from build123d import *

# Parameters (mm, degrees)
CYLINDER001_R     = 8.4
CYLINDER001_DEPTH = 5.5
CYLINDER004_R     = 7.2
CYLINDER004_DEPTH = 6.5
CYLINDER003_R     = 10.4
CYLINDER003_DEPTH = 1
CYLINDER002_R     = 10.4
CYLINDER002_DEPTH = 2.75
SKETCH013_R       = 9.6
SKETCH013_R_2     = 2.2
PAD011_DEPTH      = 3.75


with BuildPart() as bearing_holder_extract:
    # Cylinder001 → Cylinder001 (new body)
    with BuildSketch(Plane.XY):
        Circle(CYLINDER001_R)
    extrude(amount=CYLINDER001_DEPTH)


with BuildPart() as bearing_holder_extract_fusion:
    # Cylinder004 → Cylinder004 (new body)
    with BuildSketch(Plane.XY.offset(-1)):
        Circle(CYLINDER004_R)
    extrude(amount=CYLINDER004_DEPTH)

    # Fusion001: union bearing holder extract
    add(bearing_holder_extract.part)


with BuildPart() as bearing_holder_disk:
    # Cylinder003 → Cylinder003 (new body)
    with BuildSketch(Plane.XY.offset(-1)):
        Circle(CYLINDER003_R)
    extrude(amount=CYLINDER003_DEPTH)


with BuildPart() as bearing_holder_body:
    # Cylinder002 → Cylinder002 (new body)
    with BuildSketch(Plane.XY):
        Circle(CYLINDER002_R)
    extrude(amount=CYLINDER002_DEPTH)

    # Fusion002: union bearing holder disk
    add(bearing_holder_disk.part)

    # Cut003: cut bearing holder extract fusion
    add(bearing_holder_extract_fusion.part, mode=Mode.SUBTRACT)


with BuildPart() as bearing_holder_body_1:
    # Cut003 placement: moved
    add(bearing_holder_body.part.moved(Location((0, 0, 1))))


with BuildPart() as bearing_holder_body_clone:
    # Body009 base: copy of bearing holder body
    add(bearing_holder_body_1.part)


with BuildPart() as bearing_holder_body_clone_1:
    # Clone002 placement: moved
    add(bearing_holder_body_clone.part.moved(Location((0, 0, -1))))


with BuildPart() as bearing_holder_body_clone_2:
    # Body009 placement: moved
    add(bearing_holder_body_clone_1.part.moved(Location((10, 25, 1))))


with BuildPart() as bearing_holder_body_clone001:
    # Body010 base: copy of bearing holder body
    add(bearing_holder_body_1.part)


with BuildPart() as bearing_holder_body_clone001_1:
    # Clone003 placement: moved
    add(bearing_holder_body_clone001.part.moved(Location((0, 0, -1))))


with BuildPart() as bearing_holder_body_clone001_2:
    # Body010 placement: moved
    add(bearing_holder_body_clone001_1.part.moved(Location((-26, -20, 1))))


with BuildPart() as bearing_holder_body_clone002:
    # Body011 base: copy of bearing holder body
    add(bearing_holder_body_1.part)


with BuildPart() as bearing_holder_body_clone002_1:
    # Clone004 placement: moved
    add(bearing_holder_body_clone002.part.moved(Location((0, 0, -1))))


with BuildPart() as bearing_holder_body_clone002_2:
    # Body011 placement: moved
    add(bearing_holder_body_clone002_1.part.moved(Location((46, -20, 1))))


with BuildPart() as top_bearing_plate_fusion_clone:
    # Sketch013 → Pad011 (new body)
    with BuildSketch(Plane.XY):
        with BuildLine():
            Line((1.646601, 32.001411), (-34.644004, -12.858892))
            ThreePointArc((-34.644004, -12.858892), (-36.048496, -24.763041), (-25.91021, -31.158079))
            Line((-25.91021, -31.158079), (45.861431, -31.158079))
            ThreePointArc((45.861431, -31.158079), (55.920577, -24.833853), (54.581009, -13.027591))
            Line((54.581009, -13.027591), (18.635324, 31.950884))
            ThreePointArc((18.635324, 31.950884), (10.153066, 36.045837), (1.646601, 32.001411))
        make_face()
        with Locations((-25.91021, -19.924263)):
            Circle(SKETCH013_R, mode=Mode.SUBTRACT)
        with Locations((10.120649, 25.146166)):
            Circle(SKETCH013_R, mode=Mode.SUBTRACT)
        with Locations((45.861431, -19.996062)):
            Circle(SKETCH013_R, mode=Mode.SUBTRACT)
        with Locations((-11.219142, 6.834813)):
            Circle(SKETCH013_R_2, mode=Mode.SUBTRACT)
        with Locations((10.016696, -25.022005)):
            Circle(SKETCH013_R_2, mode=Mode.SUBTRACT)
        with Locations((31.129337, 6.879182)):
            Circle(SKETCH013_R_2, mode=Mode.SUBTRACT)
    extrude(amount=PAD011_DEPTH)

    # Fusion003: union bearing holder body clone, bearing holder body clone001, bearing holder body clone002
    add(bearing_holder_body_clone_2.part)
    add(bearing_holder_body_clone001_2.part)
    add(bearing_holder_body_clone002_2.part)


with BuildPart() as top_bearing_plate_fusion_clone_1:
    # Body021 placement: moved
    add(top_bearing_plate_fusion_clone.part.moved(Location((-10, -8, 0))))


solid = top_bearing_plate_fusion_clone_1.part
For this review, take the finished solid that the model builds, in its own axes (mm). A direction names the side the tool comes from. Round coordinates to 2 decimals unless told otherwise and drop trailing zeros. Write each loop counter-clockwise with the first axis right and the second up, starting at its lowest first coordinate (ties: lowest second). Pieces come first, ordered by that corner, then holes. Notation, with made-up numbers: (75.25, 66.25) - (123.25, 66.25) arc R13 ccw to (123.25, 75.25) - close; hole circle Ø10 at (-29.5, -39). An arc over 180 degrees is marked (long way). Write item = value, one per line. Start each with the question number.
1. Draft analysis for pull direction X (two halves, no side actions). For faces 1 (the face through (-26.24, 1.89, 1.85)), 2 (the face through (45.843, -32.991, 1.849)), 3 (the face through (-43.193, -27.683, 0.493)), state which applies: released by +X, released by -X, zero draft, split by the parting line, or undercut.
2. Wall thickness on L1, parallel to X at y = -28, z = 2.25; L2, parallel to X at y = -28, z = 0.5; L3, parallel to X at y = -33, z = 1.55: over which ranges is each line inside the solid? List them lowest first.
3. For faces 4 (the face through (18.93, -1.02, 1.85)), 5 (the face through (-29, -25, 1)), list the 3-axis set-ups (+Z, -Z, +X, -X, +Y, -Y) from which the entire face can be reached by the end or side of a thin tool; tool diameter is ignored.
4. For pin 1 Ø16.5 at (x, y) = (0, 17) entering from +Z; pin 2 Ø11.5 at (x, y) = (36, -28) entering from -Z, all flat-tipped, find the tip position at first contact; note any pin that passes through.
5. Consider section A-A on x = -33. State the section outline as (y, z) points, plus the area to 3 significant figures.
6. Consider section C-C on x = 0. State the section outline as (y, z) points, plus the area to 3 significant figures.
7. Consider section B-B on y = 13. State the section outline as (x, z) points.
8. Consider section D-D on z = 2.7. State the section outline as (x, y) points, plus the area to 3 significant figures.
Evaluation:
q1.face_1 = released by -X
q1.face_2 = released by +X
q1.face_3 = undercut
q2.L1 = -47.14 to -44.4, -27.6 to 27.6, 44.4 to 47.02
q2.L2 = -47.14 to -43.2, -28.8 to 28.8, 43.2 to 47.02
q2.L3 = -45.93 to -42.75, -29.25 to -2.18, 2.22 to 29.25, 42.75 to 45.84
q3.face_4 = +Z, -Z
q3.face_5 = +Z
q4.pin_1 = 1
q4.pin_2 = through
q5.outline = (-39.16, 0) - (-34.55, 0) - (-34.55, 1) - (-35.85, 1) - (-35.85, 3.75) - (-39.16, 3.75) - close; (-21.45, 0) - (-6.47, 0) - (-6.47, 3.75) - (-20.15, 3.75) - (-20.15, 1) - (-21.45, 1) - close
q5.area = 66.4 mm2
q6.outline = (-39.16, 0) - (-35.22, 0) - (-35.22, 3.75) - (-39.16, 3.75) - close; (-30.82, 0) - (9.8, 0) - (9.8, 1) - (8.6, 1) - (8.6, 3.75) - (-30.82, 3.75) - close; (24.2, 0) - (28.05, 0) - (28.05, 3.75) - (25.4, 3.75) - (25.4, 1) - (24.2, 1) - close
q6.area = 175 mm2
q7.outline = (-17.25, 0) - (-5.99, 0) - (-5.99, 1) - (-7.39, 1) - (-7.39, 3.75) - (-17.25, 3.75) - close; (5.99, 0) - (17.39, 0) - (17.39, 3.75) - (7.39, 3.75) - (7.39, 1) - (5.99, 1) - close
q8.outline = (-44.64, -20.86) arc R11.23 ccw to (-35.91, -39.16) - (35.86, -39.16) arc R11.16 ccw to (44.58, -21.03) - (8.64, 23.95) arc R10.9 ccw to (-8.35, 24) - close; hole circle Ø16.8 at (-36, -28); hole circle Ø4.4 at (-21.22, -1.17); hole circle Ø16.8 at (0, 17); hole circle Ø4.4 at (0.02, -33.02); hole circle Ø4.4 at (21.13, -1.12); hole circle Ø16.8 at (36, -28)
q8.area = 3,370 mm2
